from build123d import *

# Parameters (mm, degrees)
BOSS_EXTRUDE1_DEPTH = 6.35
SKETCH2_W           = 20
SKETCH2_H           = 2.5
BOSS_EXTRUDE2_DEPTH = 6.35
SKETCH4_W           = 7
SKETCH4_H           = 2.3
BOSS_EXTRUDE3_DEPTH = 6.35
SKETCH5_W           = 0.45
SKETCH5_H           = 23.7
CUT_EXTRUDE1_DEPTH  = 10


with BuildPart() as part:
    # Sketch1 → Boss-Extrude1 (new body)
    with BuildSketch(Plane.XY):
        Polygon((-15.235299292, 17.883619427), (-15.235299292, 2.883619427), (-0.235299292, 2.883619427), (-0.235299292, 17.883619427), (2.264700708, 17.883619427), (2.264700708, 0.383619427), (-17.735299292, 0.383619427), (-17.735299292, 17.883619427), align=None)
    extrude(amount=BOSS_EXTRUDE1_DEPTH)

    # Sketch2 → Boss-Extrude2 (add, through all)
    with BuildSketch(Plane.XY):
        with Locations((-7.735299292, 19.133619427)):
            Rectangle(SKETCH2_W, SKETCH2_H)
    extrude(amount=BOSS_EXTRUDE2_DEPTH)

    # Sketch4 → Boss-Extrude3 (add)
    with BuildSketch(Plane.XY.offset(6.35)):
        Polygon((-17.735299292, 20.383619427), (2.264700708, 20.383619427), (2.264700708, 24.083619427), (-4.235299292, 24.083619427), (-4.235299292, 26.383619427), (-11.235299292, 26.383619427), (-11.235299292, 24.083619427), (-17.735299292, 24.083619427), align=None)
        with Locations((-7.735299292, -0.766380573)):
            Rectangle(SKETCH4_W, SKETCH4_H)
    extrude(amount=-BOSS_EXTRUDE3_DEPTH)

    # Sketch5 → Cut-Extrude1 (cut)
    with BuildSketch(Plane.XY.offset(6.35)):
        with Locations((-17.510299292, 12.233619427)):
            Rectangle(SKETCH5_W, SKETCH5_H)
    extrude(amount=-CUT_EXTRUDE1_DEPTH, mode=Mode.SUBTRACT)


solid = part.part
Design review of the part built by this model. Coordinates are the model's own, in mm. A direction names the side the tool comes from. Round coordinates to 2 decimals unless told otherwise and drop trailing zeros. Write each loop counter-clockwise with the first axis right and the second up, starting at its lowest first coordinate (ties: lowest second). Pieces come first, ordered by that corner, then holes. Notation, with made-up numbers: (-22, 60) - (-17, 60) arc R23 ccw to (-17, 95) - close; hole circle Ø9 at (51, 9.5). An arc over 180 degrees is marked (long way). Use a Markdown table: item, result. Add a question column.
1. For faces 1 (the face through (-1, 0.384, 3)), 2 (the face through (-1, 24.084, 3)), 3 (the face through (-14, 0.384, 3)), 4 (the face through (-0.235, 10, 3)), list the 3-axis set-ups (+Z, -Z, +X, -X, +Y, -Y) from which the entire face can be reached by the end or side of a thin tool; tool diameter is ignored.
2. We need section B-B (y = 5). State the section outline as (x, z) points.
3. Clearance check with flat-ended pins moving along their axes: pin 1 (4 mm diameter, centred on x = -3.5, y = 12.5, fed in from +Z); pin 2 (0.7 mm diameter, centred on y = -0.5, z = 3.5, fed in from +X); pin 3 (1.2 mm diameter, centred on y = 25, z = 2.5, fed in from -X); pin 4 (1.8 mm diameter, centred on x = -13.5, z = 3.5, fed in from +Y). State where each tip first meets the part, or that it passes through.
4. We need section D-D (x = 1). State the section outline as (y, z) points, then the cut area to 3 significant figures.
5. Mouldability with a two-part tool opening along Y and no side actions: class faces 5 (the face through (2.265, 12, 3)), 6 (the face through (-8, 2.884, 3)), 7 (the face through (-14, 24.084, 3)), 8 (the face through (-15.235, 10, 3)) as +Y half, -Y half, draft (parallel to the pull), parting line (faces both ways), or undercut.
6. We need section C-C (z = 4.75). State the section outline as (x, y) points, then the cut area to 3 significant figures.
7. We need section A-A (x = -8.5). State the section outline as (y, z) points, then the cut area to 3 significant figures.
8. Wall thickness on probe 1 along X at (y, z) = (15.5, 1); probe 2 along Y at (x, z) = (-8, 2); probe 3 along Y at (x, z) = (-13.25, 4.75): over which ranges is each line inside the solid? List them lowest first.
Output:
| question | item | result |
|---|---|---|
| 1 | face 1 | +Z, -Z, +X, -Y |
| 1 | face 2 | +Z, -Z, +X, +Y |
| 1 | face 3 | +Z, -Z, -X, -Y |
| 1 | face 4 | +Z, -Z |
| 2 | outline | (-17.29, 0) - (-15.24, 0) - (-15.24, 6.35) - (-17.29, 6.35) - close; (-0.24, 0) - (2.26, 0) - (2.26, 6.35) - (-0.24, 6.35) - close |
| 3 | pin 1 | passes through |
| 3 | pin 2 | stops at x = -4.24 |
| 3 | pin 3 | stops at x = -11.24 |
| 3 | pin 4 | stops at y = 24.08 |
| 4 | outline | (0.38, 0) - (24.08, 0) - (24.08, 6.35) - (0.38, 6.35) - close |
| 4 | area | 150 mm2 |
| 5 | face 5 | draft |
| 5 | face 6 | undercut |
| 5 | face 7 | +Y half |
| 5 | face 8 | undercut |
| 6 | outline | (-17.29, 0.38) - (-11.24, 0.38) - (-11.24, -1.92) - (-4.24, -1.92) - (-4.24, 0.38) - (2.26, 0.38) - (2.26, 24.08) - (-4.24, 24.08) - (-4.24, 26.38) - (-11.24, 26.38) - (-11.24, 24.08) - (-17.29, 24.08) - close; hole (-15.24, 2.88) - (-0.24, 2.88) - (-0.24, 17.88) - (-15.24, 17.88) - close |
| 6 | area | 271 mm2 |
| 7 | outline | (-1.92, 0) - (2.88, 0) - (2.88, 6.35) - (-1.92, 6.35) - close; (17.88, 0) - (26.38, 0) - (26.38, 6.35) - (17.88, 6.35) - close |
| 7 | area | 84.5 mm2 |
| 8 | probe 1 | x = -17.29 to -15.24, -0.24 to 2.26 |
| 8 | probe 2 | y = -1.92 to 2.88, 17.88 to 26.38 |
| 8 | probe 3 | y = 0.38 to 2.88, 17.88 to 24.08 |
